Geometry check sheet. Reference: drawing and pictorial views, mm from the part's lowest x, y, z. A direction names the side the tool comes from. Round coordinates to 2 decimals unless told otherwise and drop trailing zeros. Write each loop counter-clockwise with the first axis right and the second up, starting at its lowest first coordinate (ties: lowest second). Pieces come first, ordered by that corner, then holes. Notation, with made-up numbers: M 57.5,-2 L 67.5,-2 A19 cw 67.5,29 Z; hole C 61,86.25 d2. An arc over 180 degrees is marked long. Answer in a Markdown table with one row per item. Add a question column.
1. Go/stop test with flat-tipped pins: pin 1 Ø1.2 at (x, z) = (4, 8) entering from -Y; pin 2 Ø1.2 at (x, z) = (5, 7.5) entering from +Y; pin 3 Ø4 at (y, z) = (18, 1.5) entering from -X; pin 4 Ø1.2 at (y, z) = (2.5, 7.5) entering from +X. Record where each tip stops, or that it passes through.
2. Set-up check for the marked faces 1 and 2: record each of +Z, -Z, +X, -X, +Y, -Y from which the full face is reachable in a straight line by a thin tool's end or side.
3. Material ranges on probe 1 along Y at (x, z) = (40, 3.25); probe 2 along X at (y, z) = (28.5, 4.5); probe 3 along Z at (x, y) = (76, 44), recorded low to high.
4. Sectioned sample at C-C on z = 2.25. Record the cut outline in (x, y).
5. Sectioned sample at B-B on x = 33. Record the cut outline in (y, z).
6. Sectioned sample at D-D on y = 10.5. Record the cut outline in (x, z), plus the area to 3 significant figures.
7. Sectioned sample at A-A on z = 8.25. Record the cut outline in (x, y).
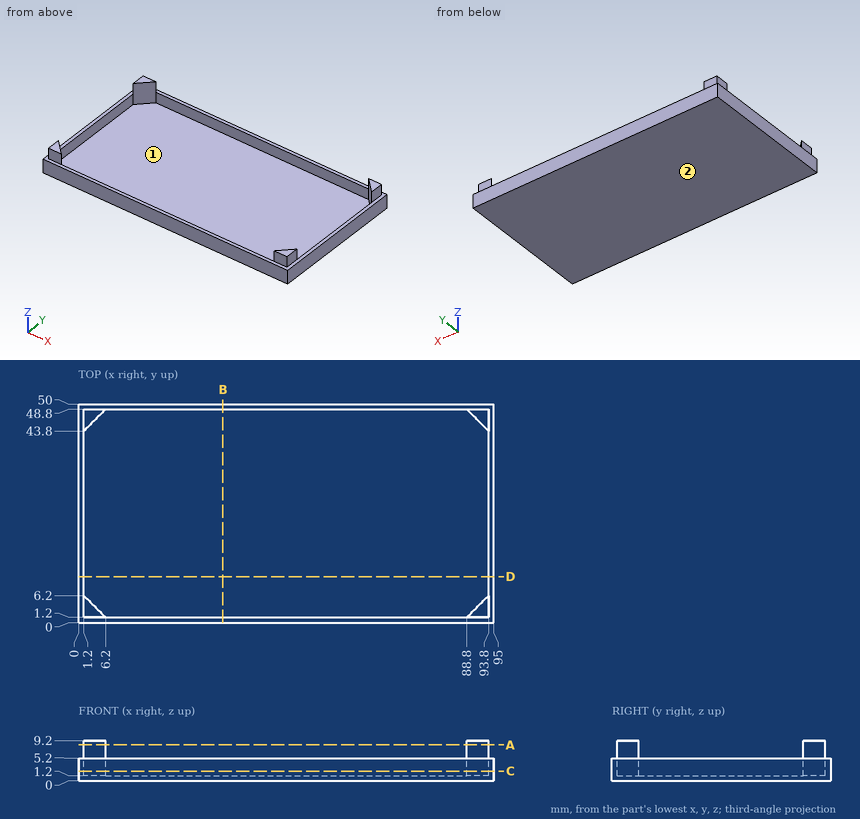
Geometry check:
| question | item | result |
|---|---|---|
| 1 | pin 1 | stops at y = 1.2 |
| 1 | pin 2 | stops at y = 48.8 |
| 1 | pin 3 | stops at x = 0 |
| 1 | pin 4 | stops at x = 93.8 |
| 2 | face 1 | +Z |
| 2 | face 2 | -Z, +X, -X, +Y, -Y |
| 3 | probe 1 | y = 0 to 1.2, 48.8 to 50 |
| 3 | probe 2 | x = 0 to 1.2, 93.8 to 95 |
| 3 | probe 3 | z = 0 to 1.2 |
| 4 | outline | M 0,0 L 95,0 L 95,50 L 0,50 Z; hole M 1.2,6.2 L 6.2,1.2 L 88.8,1.2 L 93.8,6.2 L 93.8,43.8 L 88.8,48.8 L 6.2,48.8 L 1.2,43.8 Z |
| 5 | outline | M 0,0 L 50,0 L 50,5.2 L 48.8,5.2 L 48.8,1.2 L 1.2,1.2 L 1.2,5.2 L 0,5.2 Z |
| 6 | outline | M 0,0 L 95,0 L 95,5.2 L 93.8,5.2 L 93.8,1.2 L 1.2,1.2 L 1.2,5.2 L 0,5.2 Z |
| 6 | area | 124 mm2 |
| 7 | outline | M 1.2,1.2 L 6.2,1.2 L 1.2,6.2 Z; M 1.2,43.8 L 6.2,48.8 L 1.2,48.8 Z; M 88.8,1.2 L 93.8,1.2 L 93.8,6.2 Z; M 88.8,48.8 L 93.8,43.8 L 93.8,48.8 Z |
